Answer from the drawing. Dimensions are ordinates in mm from the lowest x, y and z of the part. Round coordinates to 2 decimals unless told otherwise and drop trailing zeros. Loops run counter-clockwise (first coordinate to the right, second up) from the corner with the lowest first, then second, coordinate; pieces in that order, holes last.
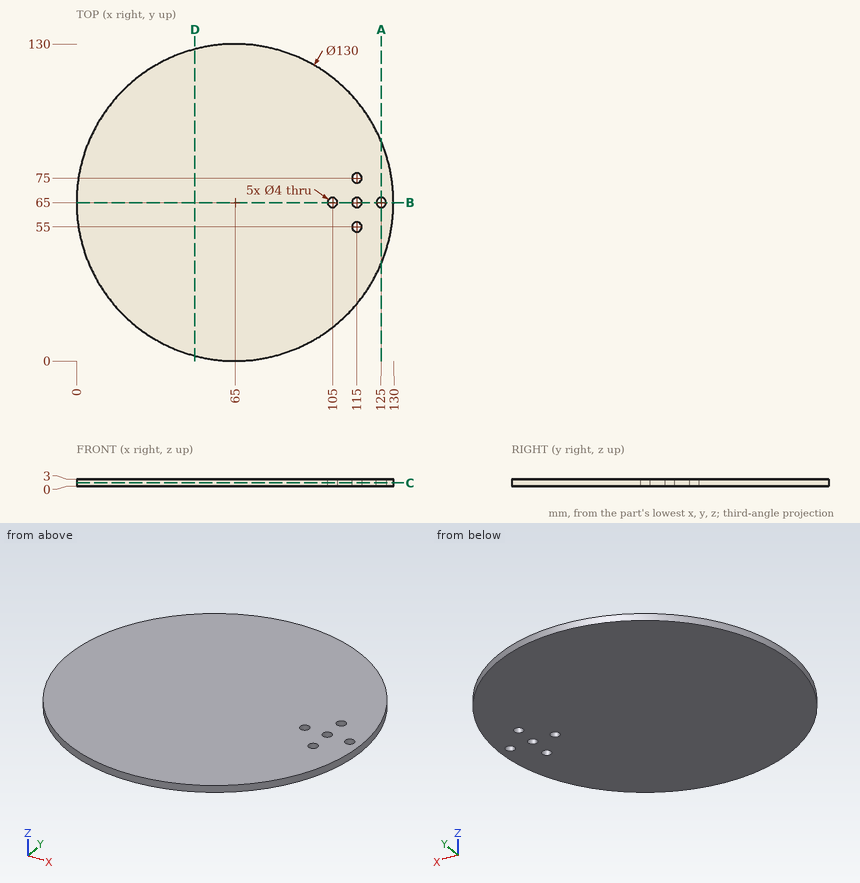
Item 1: Section C-C, the plane z = 1.4 is taken. Give the vertices of the cut face in (x, y).
Item 2: Section D-D, the plane x = 48.5 is taken. Give the vertices of the cut face in (y, z), plus the area to 3 significant figures.
Item 3: Straight lines are drawn through the part: line 1 (X direction, y = 66, z = 0.75); line 2 (Y direction, x = 115, z = 2.05); line 3 (X direction, y = 56, z = 1.7). For each, find the intervals that lie inside material, in ascending order.
Item 4: Section B-B, the plane y = 65 is taken. Give the vertices of the cut face in (x, z).
Item 5: Section A-A, the plane x = 125 is taken. Give the vertices of the cut face in (y, z).
Item 6: This flat-tipped pin is pushed along its axis until it touches: P1, Ø1, axis at x = 105.5, z = 0.5, coming from the +Y side. Where does it stop, or does it pass through?
Answer below:
1. outline: circle Ø130 at (65, 65); hole circle Ø4 at (105, 65); hole circle Ø4 at (115, 55); hole circle Ø4 at (115, 65); hole circle Ø4 at (115, 75); hole circle Ø4 at (125, 65)
2. outline: (2.13, 0) - (127.87, 0) - (127.87, 3) - (2.13, 3) - close
2. area: 377 mm2
3. line 1: x = 0.01 to 103.27, 106.73 to 113.27, 116.73 to 123.27, 126.73 to 129.99
3. line 2: y = 23.47 to 53, 57 to 63, 67 to 73, 77 to 106.53
3. line 3: x = 0.63 to 113.27, 116.73 to 129.37
4. outline: (0, 0) - (103, 0) - (103, 3) - (0, 3) - close; (107, 0) - (113, 0) - (113, 3) - (107, 3) - close; (117, 0) - (123, 0) - (123, 3) - (117, 3) - close; (127, 0) - (130, 0) - (130, 3) - (127, 3) - close
5. outline: (40, 0) - (63, 0) - (63, 3) - (40, 3) - close; (67, 0) - (90, 0) - (90, 3) - (67, 3) - close
6. P1: stops at y = 116.23
